from build123d import *

# Parameters (mm, degrees)
ESBO_O2_R                = 4.5
RESSALTO_EXTRUS_O1_DEPTH = 1
ESBO_O3_R                = 1.125
RESSALTO_EXTRUS_O2_DEPTH = 3
ESBO_O4_R                = 4.5
ESBO_O4_R_2              = 2.3
RESSALTO_EXTRUS_O3_DEPTH = 3


with BuildPart() as part:
    # Esboço2 → Ressalto-extrusão1 (new body)
    with BuildSketch(Plane.XY):
        Circle(ESBO_O2_R)
    extrude(amount=RESSALTO_EXTRUS_O1_DEPTH)

    # Esboço3 → Ressalto-extrusão2 (add)
    with BuildSketch(Plane(origin=(0, 0, 0), x_dir=(-1, 0, 0), z_dir=(0, 0, -1))):
        Circle(ESBO_O3_R)
    extrude(amount=RESSALTO_EXTRUS_O2_DEPTH)

    # Esboço4 → Ressalto-extrusão3 (add)
    with BuildSketch(Plane.XY.offset(1)):
        Circle(ESBO_O4_R)
        Circle(ESBO_O4_R_2, mode=Mode.SUBTRACT)
    extrude(amount=RESSALTO_EXTRUS_O3_DEPTH)


solid = part.part
The model under review builds one solid part; all positions refer to its coordinate system, in mm. A direction names the side the tool comes from. Give positions to 0.01 mm unless a question says otherwise; leave off trailing zeros. Order: outer loops, then holes, each group sorted by start corner. A loop starts at its lowest first (then second) coordinate and runs counter-clockwise, first axis right, second up. Notation, with made-up numbers: (5, 5) -> (31, 5) arc R15 cw to (31, 9) -> close; hole circle Ø2 at (54, 61). An arc over 180 degrees is marked (long way). Write item = value, one per line. Start each with the question number.
(1) Take a section at D-D (z = -0.75). Write out the cut boundary in (x, y) (3 decimals).
(2) Tool access review of faces 5 (the cylindrical face through (-0.59, 4.46, 1.97)), 6 (the flat face through (1, -1, 0)): name each direction out of +Z, -Z, +X, -X, +Y, -Y from which nothing blocks a thin tool from reaching the whole face with its end or side.
(3) For pin 1 Ø4.5 at (x, y) = (-2, -2) entering from -Z; pin 2 Ø1.5 at (y, z) = (1.5, -1.5) entering from -X; pin 3 Ø1 at (x, y) = (-2.5, -1) entering from -Z; pin 4 Ø4 at (x, y) = (0, 0) entering from +Z, all flat-tipped, find the tip position at first contact; note any pin that passes through.
(4) Take a section at C-C (z = 1.5). Write out the cut boundary in (x, y).
(5) For L1, parallel to Y at x = 0, z = 3.25; L2, parallel to Z at x = 3.25, y = -0.25; L3, parallel to X at y = 0.5, z = 1.25 (3 decimals), list the stretches that pass through material, from the lowest coordinate up. Write a range as from..to.
(6) Draft analysis for pull direction Y (two halves, no side actions). For faces 1 (the flat face through (0, 0, -3)), 2 (the flat face through (0, 0, 1)), 3 (the cylindrical face through (-1.825, -1.4, 2.479)), 4 (the cylindrical face through (0.146, 1.115, -1.479)), state which applies: +Y half, -Y half, draft (parallel to the pull), parting line (faces both ways), or undercut.
(7) Take a section at A-A (y = 0). Write out the cut boundary in (x, z) (3 decimals), plus the area to 4 significant figures.
Returned:
q1.outline = circle Ø2.25 at (0, 0)
q2.face_5 = +Z, -Z
q2.face_6 = -Z
q3.pin_1 = -3
q3.pin_2 = -0.84
q3.pin_3 = 0
q3.pin_4 = 1
q4.outline = circle Ø9 at (0, 0); hole circle Ø4.6 at (0, 0)
q5.L1 = -4.5..-2.3, 2.3..4.5
q5.L2 = 0..4
q5.L3 = -4.472..-2.245, 2.245..4.472
q6.face_1 = draft
q6.face_2 = undercut
q6.face_3 = undercut
q6.face_4 = parting line
q7.outline = (-4.5, 0) -> (-1.125, 0) -> (-1.125, -3) -> (1.125, -3) -> (1.125, 0) -> (4.5, 0) -> (4.5, 4) -> (2.3, 4) -> (2.3, 1) -> (-2.3, 1) -> (-2.3, 4) -> (-4.5, 4) -> close
q7.area = 28.95 mm²
